```python
from build123d import *

# Parameters (mm, degrees)
CABCAPOUTLINE_THICKNESS_DEPTH = 17.78
SKETCH3_W                     = 44.45
SKETCH3_H                     = 17.78
CAPBACKLEDGE_DEPTH_DEPTH      = 5.08
CABSIDELEDGECUTS_W            = 17.78
CABSIDELEDGECUTS_H            = 177.363711221
CABSIDELEDGE_DEPTH_DEPTH      = 9.525
SKETCH5_R                     = 1.5875
SKETCH5_R_2                   = 3.302
CUT_EXTRUDE3_DEPTH            = 17.78


with BuildPart() as part:
    # CabCapOutline → CabCapOutline_Thickness (new body)
    with BuildSketch(Plane.XY):
        Polygon((12324.291666666, -6347.976211221), (12324.291666666, -6170.6125), (12279.841666666, -6170.6125), (12279.841666666, -6188.3925), (12197.291666666, -6188.3925), (12197.291666666, -6292.5325), (11822.641666666, -6292.5325), (11822.641666666, -6188.3925), (11740.091666666, -6188.3925), (11740.091666666, -6170.6125), (11695.641666666, -6170.6125), (11695.641666666, -6347.976211221), align=None)
    extrude(amount=-CABCAPOUTLINE_THICKNESS_DEPTH)

    # Sketch3 → CapBackLedge_Depth (cut)
    with BuildSketch(Plane.XY):
        with Locations((11717.866666666, -6179.5025)):
            Rectangle(SKETCH3_W, SKETCH3_H)
        with Locations((12302.066666666, -6179.5025)):
            Rectangle(SKETCH3_W, SKETCH3_H)
    extrude(amount=-CAPBACKLEDGE_DEPTH_DEPTH, mode=Mode.SUBTRACT)

    # CabSideLedgeCuts → CabSideLedge_Depth (cut)
    with BuildSketch(Plane.XY):
        with Locations((11704.531666666, -6259.294355611)):
            Rectangle(CABSIDELEDGECUTS_W, CABSIDELEDGECUTS_H)
        with Locations((12315.401666666, -6259.294355611)):
            Rectangle(CABSIDELEDGECUTS_W, CABSIDELEDGECUTS_H)
    extrude(amount=-CABSIDELEDGE_DEPTH_DEPTH, mode=Mode.SUBTRACT)

    # Sketch5 → Cut-Extrude3 (cut)
    with BuildSketch(Plane.XY):
        with Locations((11704.531666666, -6316.444355611)):
            Circle(SKETCH5_R)
        with Locations((11704.531666666, -6259.294355611)):
            Circle(SKETCH5_R)
        with Locations((11704.531666666, -6202.144355611)):
            Circle(SKETCH5_R)
        with Locations((11726.756666666, -6179.5025)):
            Circle(SKETCH5_R)
        with Locations((11748.981666666, -6208.7125)):
            Circle(SKETCH5_R)
        with Locations((11748.981666666, -6272.2125)):
            Circle(SKETCH5_R)
        with Locations((11825.181666666, -6301.4225)):
            Circle(SKETCH5_R)
        with Locations((11948.371666666, -6301.4225)):
            Circle(SKETCH5_R)
        with Locations((12071.561666666, -6301.4225)):
            Circle(SKETCH5_R)
        with Locations((12194.751666666, -6301.4225)):
            Circle(SKETCH5_R)
        with Locations((12315.401666666, -6316.444355611)):
            Circle(SKETCH5_R)
        with Locations((12315.401666666, -6259.294355611)):
            Circle(SKETCH5_R)
        with Locations((12270.951666666, -6272.2125)):
            Circle(SKETCH5_R)
        with Locations((12270.951666666, -6208.7125)):
            Circle(SKETCH5_R)
        with Locations((12315.401666666, -6202.144355611)):
            Circle(SKETCH5_R)
        with Locations((12293.176666666, -6179.5025)):
            Circle(SKETCH5_R)
        with Locations((11742.336730696, -6186.14743597)):
            Circle(SKETCH5_R_2)
        with Locations((12277.596602636, -6186.14743597)):
            Circle(SKETCH5_R_2)
    extrude(amount=-CUT_EXTRUDE3_DEPTH, mode=Mode.SUBTRACT)


solid = part.part
```
Design review of the part built by this model. Coordinates are the model's own, in mm. A direction names the side the tool comes from. Coordinates: 2 decimals unless noted, no trailing zeros. Order: outer loops, then holes, each group sorted by start corner. A loop starts at its lowest first (then second) coordinate and runs counter-clockwise, first axis right, second up.
1) Clearance check with flat-ended pins moving along their axes: pin 1 (3 mm diameter, centred on x = 11748.98, y = -6208.71, fed in from +Z); pin 2 (4 mm diameter, centred on x = 12270.95, y = -6208.71, fed in from -Z); pin 3 (9 mm diameter, centred on x = 11724.5, y = -6177, fed in from +Z); pin 4 (1.5 mm diameter, centred on y = -6330, z = -5.5, fed in from +X). State where each tip first meets the part, or that it passes through.
2) Take a section at D-D, the plane x = 12205.5. Give the boundary of the cut face in (y, z), and give its area (3 significant figures).
3) Take a section at B-B, the plane y = -6324.5. Give the boundary of the cut face in (x, z) (3 decimals).
4) For faces 3 (the flat face through (11727, -6177, -5.08)), 4 (the flat face through (12317, -6258, -9.525)), 5 (the flat face through (12006, -6303, 0)), 6 (the flat face through (12236, -6188.392, -9)), 7 (the flat face through (11706, -6258, -9.525)), list the 3-axis set-ups (+Z, -Z, +X, -X, +Y, -Y) from which the entire face can be reached by the end or side of a thin tool; tool diameter is ignored.
5) Take a section at A-A, the plane y = -6281. Give the boundary of the cut face in (x, z) (3 decimals).
6) Wall thickness on line 1 along X through (y, z) = (-6264.5, -9); line 2 along X through (y, z) = (-6272.5, -11); line 3 along X through (y, z) = (-6205, -11.75): over which ranges is each line inside the solid? List them lowest first.
7) Take a section at C-C, the plane x = 12058.5. Give the boundary of the cut face in (y, z).
8) Mouldability with a two-part tool opening along X and no side actions: class faces 1 (the flat face through (11822.642, -6241, -9)), 2 (the flat face through (12006, -6347.976, -9)) as +X half, -X half, draft (parallel to the pull), parting line (faces both ways), or undercut.
Returned:
1. pin 1: passes through
1. pin 2: stops at z = -17.78
1. pin 3: stops at z = -5.08
1. pin 4: stops at x = 12306.51
2. outline: (-6347.98, -17.78) - (-6188.39, -17.78) - (-6188.39, 0) - (-6347.98, 0) - close
2. area: 2,840 mm2
3. outline: (11695.642, -17.78) - (12324.292, -17.78) - (12324.292, -9.525) - (12306.512, -9.525) - (12306.512, 0) - (11713.422, 0) - (11713.422, -9.525) - (11695.642, -9.525) - close
4. face 3: +Z, +X, -X, +Y
4. face 4: +Z, +X, +Y, -Y
4. face 5: +Z, +X, -X, +Y, -Y
4. face 6: +Z, -Z, +Y
4. face 7: +Z, -X, +Y, -Y
5. outline: (11695.642, -17.78) - (11822.642, -17.78) - (11822.642, 0) - (11713.422, 0) - (11713.422, -9.525) - (11695.642, -9.525) - close; (12197.292, -17.78) - (12324.292, -17.78) - (12324.292, -9.525) - (12306.512, -9.525) - (12306.512, 0) - (12197.292, 0) - close
6. line 1: x = 11713.42 to 11822.64, 12197.29 to 12306.51
6. line 2: x = 11695.64 to 11747.42, 11750.54 to 11822.64, 12197.29 to 12269.39, 12272.51 to 12324.29
6. line 3: x = 11695.64 to 11822.64, 12197.29 to 12324.29
7. outline: (-6347.98, -17.78) - (-6292.53, -17.78) - (-6292.53, 0) - (-6347.98, 0) - close
8. face 1: undercut
8. face 2: draft
